Part model, mm, in its own coordinate system. A direction names the side the tool comes from. Coordinates: 2 decimals unless noted, no trailing zeros. Write each loop counter-clockwise with the first axis right and the second up, starting at its lowest first coordinate (ties: lowest second). Pieces come first, ordered by that corner, then holes. Notation, with made-up numbers: M 8.25,54.5 L 21.25,54.5 A21 ccw 21.25,61.5 Z; hole C -28.5,-26 d1. An arc over 180 degrees is marked long. Use a Markdown table: item, result. Add a question column.
Q1. Slice it at A-A on z = 16. Write the cut outline in (x, y).
Q2. Tool access for faces 4 (the flat face through (-7, -58, 7)), 5 (the flat face through (7.01, -54.29, 24.49)), 6 (the flat face through (-15, -19, -10)), 7 (the flat face through (7.29, -54.01, -24.49)), 8 (the cylindrical face through (-14.965, -38.752, -14.287)): list every direction of +Z, -Z, +X, -X, +Y, -Y with a clear straight run to the whole face (end or side of a thin tool).
Q3. Pin check, flat tips, straight feed: pin 1 Ø1 at (y, z) = (-51, -16) entering from +X; pin 2 Ø1.5 at (x, z) = (-15.5, 5.5) entering from +Y; pin 3 Ø9 at (y, z) = (-21.5, 2) entering from -X. Stop position of each tip, or through.
Q4. Mould opens along Y. For faces 1 (the flat face through (-15, -38, -11)), 2 (the cylindrical face through (0.2, -46.5, 4.9)), 3 (the flat face through (0, -32, 24.995)) say: released by +Y, released by -Y, zero draft, split by the parting line, or undercut.
Q5. Slice it at C-C on y = -55. Write the cut outline in (x, z) (3 decimals).
Q6. Slice it at D-D on y = -7. Write the cut outline in (x, z) (3 decimals).
Q7. Wall check: L1, parallel to Z at x = -14.5, y = -56.5 (3 decimals); L2, parallel to Z at x = -14, y = -31 (3 decimals); L3, parallel to X at y = -36, z = 4.5. Give the ranges that are in metal, low to high. Write a range as from..to.
from build123d import *

# Parameters (mm, degrees)
SKETCH1_W           = 35
SKETCH1_H           = 49.99
BOSS_EXTRUDE1_DEPTH = 64.5
CUT_EXTRUDE1_REACH  = 85.46
CUT_EXTRUDE2_REACH  = 79.524
SKETCH3_W           = 14
SKETCH3_H           = 20
FILLET1_R           = 7
SKETCH4_W           = 5
SKETCH4_H           = 20
CUT_EXTRUDE3_DEPTH  = 43
SKETCH5_W           = 30
SKETCH5_H           = 5
CUT_EXTRUDE4_DEPTH  = 5
FILLET5_R           = 2.5
FILLET6_R           = 2.5
CHAMFER1_SIZE       = 1


with BuildPart() as part:
    # Sketch1 → Boss-Extrude1 (new body)
    with BuildSketch(Plane(origin=(0, 0, 0), x_dir=(1, 0, 0), z_dir=(0, 1, 0))):
        Rectangle(SKETCH1_W, SKETCH1_H)
    extrude(amount=-BOSS_EXTRUDE1_DEPTH)

    # Sketch2 → Cut-Extrude1 (cut, up to next)
    with BuildSketch(Plane.XY.offset(24.995), mode=Mode.PRIVATE) as cut_extrude1_sk1:
        Polygon((-2.5, -64.5), (17.5, -44.5), (17.5, -64.5), align=None)
    cut_extrude1_tool1 = extrude(cut_extrude1_sk1.sketch, amount=-CUT_EXTRUDE1_REACH, mode=Mode.PRIVATE) & part.part
    add(cut_extrude1_tool1.solids().sort_by_distance((10.833333, -57.833333, 24.995))[0], mode=Mode.SUBTRACT)

    # Sketch3 → Cut-Extrude2 (cut, up to next)
    with BuildSketch(Plane.ZY.offset(17.5), mode=Mode.PRIVATE) as cut_extrude2_sk1:
        with Locations((0, -54.5)):
            Rectangle(SKETCH3_W, SKETCH3_H)
    cut_extrude2_tool1 = extrude(cut_extrude2_sk1.sketch, amount=-CUT_EXTRUDE2_REACH, mode=Mode.PRIVATE) & part.part
    add(cut_extrude2_tool1.solids().sort_by_distance((-17.5, -54.5, 0))[0], mode=Mode.SUBTRACT)

    # Fillet1
    fillet1_edges = [part.edges().sort_by_distance(p)[0] for p in [
        (0, -44.5, -7),
        (0, -44.5, 7),
    ]]
    fillet(fillet1_edges, radius=FILLET1_R - 0.0001)  # a hair under: the kernel refuses the full size

    # Sketch4 → Cut-Extrude3 (cut)
    with BuildSketch(Plane(origin=(0, 0, 0), x_dir=(1, 0, 0), z_dir=(0, 1, 0))):
        with Locations((-15, 0)):
            Rectangle(SKETCH4_W, SKETCH4_H)
    extrude(amount=-CUT_EXTRUDE3_DEPTH, mode=Mode.SUBTRACT)

    # Sketch5 → Cut-Extrude4 (cut)
    with BuildSketch(Plane.ZY.offset(17.5)):
        with Locations((0, -40.5)):
            Rectangle(SKETCH5_W, SKETCH5_H)
    extrude(amount=-CUT_EXTRUDE4_DEPTH, mode=Mode.SUBTRACT)

    # Fillet5
    fillet5_edges = [part.edges().sort_by_distance(p)[0] for p in [
        (-15, -38, -15),
        (-15, -43, -15),
    ]]
    fillet(fillet5_edges, radius=FILLET5_R - 0.0001)  # a hair under: the kernel refuses the full size

    # Fillet6
    fillet6_edges = [part.edges().sort_by_distance(p)[0] for p in [
        (-15, -43, 15),
        (-15, -38, 15),
    ]]
    fillet(fillet6_edges, radius=FILLET6_R - 0.0001)  # a hair under: the kernel refuses the full size

    # Chamfer1
    chamfer1_edges = [part.edges().sort_by_distance(p)[0] for p in [
        (-10, -64.5, -24.995),
        (17.5, -22.25, -24.995),
        (17.5, -22.25, 24.995),
        (-10, -64.5, 24.995),
        (7.5, -54.5, -24.995),
        (7.5, -54.5, 24.995),
        (0, 0, 24.995),
        (-17.5, 0, -17.4975),
        (-17.5, 0, 17.4975),
        (0, 0, -24.995),
        (17.5, 0, 0),
        (-15, 0, 10),
        (-12.5, 0, 0),
        (-15, 0, -10),
        (-17.5, -32.25, 24.995),
        (-17.5, -32.25, -24.995),
    ]]
    chamfer(chamfer1_edges, length=CHAMFER1_SIZE)


solid = part.part
Recorded:
| question | item | result |
|---|---|---|
| 1 | outline | M -17.5,-64.5 L -2.5,-64.5 L 17.5,-44.5 L 17.5,-1 L 16.5,0 L -16.5,0 L -17.5,-1 Z |
| 2 | face 4 | +X, -X, -Y |
| 2 | face 5 | +Z, +X, -Y |
| 2 | face 6 | -X, +Y |
| 2 | face 7 | -Z, +X, -Y |
| 2 | face 8 | -X |
| 3 | pin 1 | x = 11.5 |
| 3 | pin 2 | y = -43 |
| 3 | pin 3 | x = -12.5 |
| 4 | face 1 | undercut |
| 4 | face 2 | released by -Y |
| 4 | face 3 | zero draft |
| 5 | outline | M -17.5,-23.995 L -16.5,-24.995 L 5.586,-24.995 L 7,-23.995 L 7,-7 L -17.5,-7 Z; M -17.5,7 L 7,7 L 7,23.995 L 5.586,24.995 L -16.5,24.995 L -17.5,23.995 Z |
| 6 | outline | M -17.5,-23.995 L -16.5,-24.995 L 16.5,-24.995 L 17.5,-23.995 L 17.5,23.995 L 16.5,24.995 L -16.5,24.995 L -17.5,23.995 L -17.5,10 L -12.5,10 L -12.5,-10 L -17.5,-10 Z |
| 7 | L1 | -24.995..-7, 7..24.995 |
| 7 | L2 | -24.995..-10, 10..24.995 |
| 7 | L3 | -12.5..17.5 |
